Build history of the part. All positions in model axes, mm. Face numbers are marked on the shaded views. A direction names the side the tool comes from. Round coordinates to 2 decimals unless told otherwise and drop trailing zeros. Write each loop counter-clockwise with the first axis right and the second up, starting at its lowest first coordinate (ties: lowest second). Pieces come first, ordered by that corner, then holes. Notation, with made-up numbers: (18, -35) -> (42, -35) arc R28 cw to (42, -9) -> close; hole circle Ø5 at (-39, 74.25). An arc over 180 degrees is marked (long way). Answer in a Markdown table with one row per item.
```python
from build123d import *

# Parameters (mm, degrees)
SKETCH_W        = 53
SKETCH_H        = 37.5
SKETCH_W_2      = 49
SKETCH_H_2      = 33.5
PAD_DEPTH       = 32
SKETCH001_W     = 53
SKETCH001_H     = 37.5
PAD001_DEPTH    = 2
SKETCH002_W     = 53
SKETCH002_H     = 37.5
PAD002_DEPTH    = 2
SKETCH003_W     = 33.5
SKETCH003_H     = 32
POCKET_DEPTH    = 2
SKETCH004_W     = 10
SKETCH004_H     = 5.75
SKETCH004_W_2   = 12.5
SKETCH004_W_3   = 9.9999999999
POCKET001_DEPTH = 5
SKETCH005_W     = 51
SKETCH005_H     = 1.8
SKETCH005_H_2   = 1.5
PAD003_DEPTH    = 33.5
SKETCH006_W     = 30.5
SKETCH006_H     = 9
POCKET002_DEPTH = 51
SKETCH007_W     = 17.616245
SKETCH007_H     = 6
PAD004_DEPTH    = 5
SKETCH008_R     = 0.8
POCKET003_DEPTH = 5
SKETCH009_W     = 17.616245
SKETCH009_H     = 6
PAD005_DEPTH    = 3.5
SKETCH010_R     = 0.8
POCKET004_DEPTH = 6
CHAMFER_SIZE    = 3.499
CHAMFER001_SIZE = 4.99
FILLET_R        = 1.99
SKETCH012_W     = 53
SKETCH012_H     = 4
PAD006_DEPTH    = 6
FILLET001_R     = 5
SKETCH013_W     = 6
SKETCH013_H     = 5
POCKET005_DEPTH = 20
SKETCH014_W     = 9.5
SKETCH014_H     = 17
POCKET006_DEPTH = 5


with BuildPart() as part:
    # Sketch → Pad (new body)
    with BuildSketch(Plane.XY):
        Rectangle(SKETCH_W, SKETCH_H)
        Rectangle(SKETCH_W_2, SKETCH_H_2, mode=Mode.SUBTRACT)
    extrude(amount=PAD_DEPTH)

    # Sketch001 (on Face10 of Pad) → Pad001 (join)
    with BuildSketch(Plane.XY.offset(32)):
        Rectangle(SKETCH001_W, SKETCH001_H)
    extrude(amount=PAD001_DEPTH)

    # Sketch002 (on Face4 of Pad001) → Pad002 (join)
    with BuildSketch(Plane(origin=(0, 0, 0), x_dir=(1, 0, 0), z_dir=(0, 0, -1))):
        Rectangle(SKETCH002_W, SKETCH002_H)
    extrude(amount=PAD002_DEPTH)

    # Sketch003 (on Face3 of Pad002) → Pocket (cut)
    with BuildSketch(Plane.YZ.offset(26.5)):
        with Locations((0, 16)):
            Rectangle(SKETCH003_W, SKETCH003_H)
    extrude(amount=-POCKET_DEPTH, mode=Mode.SUBTRACT)

    # Sketch004 (on Face13 of Pocket) → Pocket001 (cut)
    with BuildSketch(Plane.XY.offset(34)):
        with Locations((-16.4, -10.975)):
            Rectangle(SKETCH004_W, SKETCH004_H)
        with Locations((-2.5, -10.975)):
            Rectangle(SKETCH004_W_2, SKETCH004_H)
        with Locations((11.45, -10.975)):
            Rectangle(SKETCH004_W_3, SKETCH004_H)
    extrude(amount=-POCKET001_DEPTH, mode=Mode.SUBTRACT)

    # Sketch005 (on Face36 of Pocket001) → Pad003 (join)
    with BuildSketch(Plane(origin=(0, -16.75, 0), x_dir=(-1, 0, 0), z_dir=(0, 1, 0))):
        with Locations((-1, 22.25)):
            Rectangle(SKETCH005_W, SKETCH005_H)
        with Locations((-1, 26)):
            Rectangle(SKETCH005_W, SKETCH005_H_2)
        with Locations((-1, 18.5)):
            Rectangle(SKETCH005_W, SKETCH005_H_2)
    extrude(amount=PAD003_DEPTH)

    # Sketch006 (on Face11 of Pad003) → Pocket002 (cut)
    with BuildSketch(Plane.YZ.offset(26.5)):
        with Locations((0, 22.25)):
            Rectangle(SKETCH006_W, SKETCH006_H)
    extrude(amount=-POCKET002_DEPTH, mode=Mode.SUBTRACT)

    # Sketch007 (on Face57 of Pocket002) → Pad004 (join)
    with BuildSketch(Plane.XY):
        with Locations((17.6918775, 0)):
            Rectangle(SKETCH007_W, SKETCH007_H)
    extrude(amount=PAD004_DEPTH)

    # Sketch008 (on Face24 of Pad004) → Pocket003 (cut)
    with BuildSketch(Plane.YZ.offset(26.5)):
        with Locations((0, 2.5)):
            Circle(SKETCH008_R)
    extrude(amount=-POCKET003_DEPTH, mode=Mode.SUBTRACT)

    # Sketch009 (on Face65 of Pocket003) → Pad005 (join)
    with BuildSketch(Plane(origin=(0, 0, 32), x_dir=(1, 0, 0), z_dir=(0, 0, -1))):
        with Locations((17.6918775, 0)):
            Rectangle(SKETCH009_W, SKETCH009_H)
    extrude(amount=PAD005_DEPTH)

    # Sketch010 (on Face41 of Pad005) → Pocket004 (cut)
    with BuildSketch(Plane.YZ.offset(26.5)):
        with Locations((0, 30.25)):
            Circle(SKETCH010_R)
    extrude(amount=-POCKET004_DEPTH, mode=Mode.SUBTRACT)

    # Chamfer
    chamfer_edges = [part.edges().sort_by_distance(p)[0] for p in [
        (8.883755, 0, 28.5),
    ]]
    chamfer(chamfer_edges, length=CHAMFER_SIZE)

    # Chamfer001
    chamfer001_edges = [part.edges().sort_by_distance(p)[0] for p in [
        (8.883755, 0, 5),
    ]]
    chamfer(chamfer001_edges, length=CHAMFER001_SIZE)

    # Fillet
    fillet_edges = [part.edges().sort_by_distance(p)[0] for p in [
        (0, -18.75, 34),
        (0, 18.75, 34),
        (0, 18.75, -2),
        (0, -18.75, -2),
    ]]
    fillet(fillet_edges, radius=FILLET_R)

    # Sketch012 → Pad006 (join)
    with BuildSketch(Plane.XZ.offset(18.75)):
        with Locations((0, 23.8)):
            Rectangle(SKETCH012_W, SKETCH012_H)
        with Locations((0, 8.5)):
            Rectangle(SKETCH012_W, SKETCH012_H)
    extrude(amount=PAD006_DEPTH)

    # Fillet001
    fillet001_edges = [part.edges().sort_by_distance(p)[0] for p in [
        (0, -18.75, 6.5),
        (0, -18.75, 25.8),
    ]]
    fillet(fillet001_edges, radius=FILLET001_R)

    # Sketch013 (on Face26 of Fillet001) → Pocket005 (cut)
    with BuildSketch(Plane.YZ.offset(26.5)):
        with Locations((0, 2.5)):
            Rectangle(SKETCH013_W, SKETCH013_H)
    extrude(amount=-POCKET005_DEPTH, mode=Mode.SUBTRACT)

    # Sketch014 (on Face23 of Pocket005) → Pocket006 (cut)
    with BuildSketch(Plane(origin=(0, 0, -2), x_dir=(1, 0, 0), z_dir=(0, 0, -1))):
        with Locations((10.25, -6.25)):
            Rectangle(SKETCH014_W, SKETCH014_H)
    extrude(amount=-POCKET006_DEPTH, mode=Mode.SUBTRACT)


solid = part.part
```
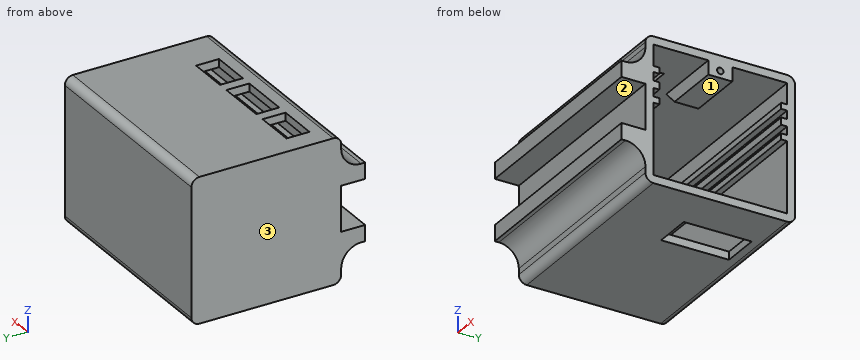
Q1. Drop flat-ended pins along their axis: P1, Ø1, axis at x = 16, z = 29.5, coming from the -Y side; P2, Ø0.6, axis at x = 13.5, z = 33, coming from the +Y side; P3, Ø0.6, axis at x = -3, z = 32.5, coming from the -Y side. Give the stop position or say it passes through.
A:
| item | result |
|---|---|
| P1 | y = -19.09 |
| P2 | y = 18.63 |
| P3 | y = -18.74 |
Q2. Saw through at C-C on z = 20.5. Write the cut outline in (x, y), plus the area to 3 significant figures.
A:
| item | result |
|---|---|
| outline | (-26.5, -18.75) -> (26.5, -18.75) -> (26.5, -16.75) -> (-24.5, -16.75) -> (-24.5, 16.75) -> (26.5, 16.75) -> (26.5, 18.75) -> (-26.5, 18.75) -> close |
| area | 279 mm² |
Q3. Which spindle directions (+Z, -Z, +X, -X, +Y, -Y) get a long thin tool onto all of the face, cutting with end or side? Do the marked faces 1, 2 and 3. Say none if no direction does.
A:
| item | result |
|---|---|
| face 1 | +X |
| face 2 | +X, -X, -Y |
| face 3 | +Z, -Z, -X, +Y, -Y |
Q4. Wall check: line 1 (Z direction, x = 24.15, y = 0); line 2 (Z direction, x = -19, y = 13); line 3 (Y direction, x = 18, z = 12). Give the ranges that are in metal, low to high. Write a range as [from, to].
A:
| item | result |
|---|---|
| line 1 | [-2, 0], [28.5, 29.45], [31.05, 34] |
| line 2 | [-2, 0], [32, 34] |
| line 3 | [-18.75, -16.75], [16.75, 18.75] |
Q5. Saw through at B-B on z = 5.5. Write the cut outline in (x, y).
A:
| item | result |
|---|---|
| outline | (-26.5, -20.75) -> (26.5, -20.75) -> (26.5, -16.75) -> (-24.5, -16.75) -> (-24.5, 16.75) -> (26.5, 16.75) -> (26.5, 18.75) -> (-26.5, 18.75) -> close |
